Autodesk Inventor part; units mm, degrees
ref_plane "XZ Plane" through (0, 0, 0) normal (0, 1, 0) x (-1, 0, 0)
ref_plane "XY Plane" through (0, 0, 0) normal (0, 0, 1) x (1, 0, 0)
sketch "Sketch1" plane through (0, 0, 0) normal (0, 0, 1) x (1, 0, 0)
  line L0 (1, -23.75) -> (1, 25.75)
  line L1 (6, 30.75) -> (37, 30.75)
  line L2 (-37, -30.75) -> (-6, -30.75)
  arc A0 (-6, -30.75) -> (1, -23.75) centre (-6, -23.75) ccw
  arc A1 (6, 30.75) -> (1, 25.75) centre (6, 25.75) ccw
  line L3 (37, 32.75) -> (6, 32.75)
  arc A2 (6, 32.75) -> (-1, 25.75) centre (6, 25.75) ccw
  line L4 (-1, 25.75) -> (-1, -23.75)
  arc A3 (-6, -28.75) -> (-1, -23.75) centre (-6, -23.75) ccw
  line L5 (-6, -28.75) -> (-37, -28.75)
  line L6 (-37, -30.75) -> (-37, -28.75)
  line L7 (37, 30.75) -> (37, 32.75)
  point P0 (0, 0)
  dimension "d5" = 30.75
  dimension "d12" = 31
  dimension "d13" = 2
sketch "Sketch2" plane through (0, 0, 0) normal (1, 0, 0) x (0, 1, 0)
  line L0 (32.75, 0) -> (32.75, -1778.57)
  arc A0 (32.75, -1778.57) -> (55.2034, -1916.4389) centre (467.25, -1778.57) ccw
  line L1 (0, 0) -> (341.65, 0)
  line L2 (55.2034, -1916.4389) -> (194.6207, -2333.1133)
  dimension "d14" = 1778.57
  dimension "d17" = 161.5
  dimension "d18" = 439.38
  dimension "d28" = 434.5
sweep "Sweep1" add profiles "Sketch1" path "Sketch2" path curves L0 A0 L2
sketch "Sketch3" plane through (1, -23.75, 0) normal (1, 0, 0) x (0, 0, -1)
  line L0 (0, 49.5) -> (0, 0)
  line L1 (0, 0) -> (1778.57, 0)
  arc A0 (1778.57, 0) -> (1934.3666, 25.3731) centre (1778.57, 491) ccw
  line L2 (1934.3666, 25.3731) -> (2351.041, 164.7904)
  line L3 (2335.3345, 211.7324) -> (2351.041, 164.7904)
  line L4 (1918.66, 72.3151) -> (2335.3345, 211.7324)
  arc A1 (1778.57, 49.5) -> (1918.66, 72.3151) centre (1778.57, 491) ccw
  line L5 (0, 49.5) -> (1778.57, 49.5)
  line L6 (50, 83.8551) -> (50, -57.0573)
  line L7 (458.25, 83.8551) -> (458.25, -57.0573)
  line L8 (653.5, 83.8551) -> (653.5, -57.0573)
  circle A2 centre (1778.57, 491) radius 467.25
  line L9 (2343.1877, 188.2614) -> (1927.8399, 48.2348)
  line L10 (2020.5284, 268.8859) -> (2149.5287, -116.6554)
  line L11 (1818.57, 100.4548) -> (1818.57, -125.8263)
  line L12 (1936.5877, 18.7348) -> (1934.3666, 25.3731)
  line L13 (1778.57, -7) -> (1778.57, 0)
  circle A3 centre (2077.4777, 98.6823) radius 10
  circle A4 centre (1818.57, 25.4653) radius 10
  circle A5 centre (653.5, 23.75) radius 10
  circle A6 centre (458.25, 23.75) radius 10
  circle A7 centre (50, 23.75) radius 10
  point P0 (0, 23.75)
  dimension "d22" = 408.25
  dimension "d23" = 195.25
  dimension "d24" = 40
  dimension "d26" = 158.977
  dimension "d29" = 20
  dimension "d30" = 20
  dimension "d31" = 20
  dimension "d32" = 20
  dimension "d33" = 20
extrude "Extrusion1" cut sketch "Sketch3" against normal blind 10 contours A7 L6 | L6 A7 | A6 L7 | L7 A6 | A5 L8 | L8 A5 | A4 L11 A2 | A2 L11 A4 | L11 A4 A2 | A2 A4 L11 | A3 L9 L10 | L10 L9 A3 | A3 L9 L10 | L10 L9 A3
sketch "Sketch4" plane through (1, -23.75, 0) normal (1, 0, 0) x (0, 0, -1)
  line L0 (2335.3345, 211.7324) -> (2333.1133, 218.3707)
  line L1 (2333.1133, 218.3707) -> (2363.5204, -278.781)
  line L2 (1778.57, -7) -> (1778.57, 0)
  line L3 (2333.1133, 218.3707) -> (2448.2703, 211.7324)
  line L4 (2448.2703, 211.7324) -> (2363.5204, -278.781)
  point P0 (0, 23.75)
  dimension "d36" = 3.5
extrude "Extrusion2" cut sketch "Sketch4" along normal through all both and the other way through all
properties part number "AAD0001149621"
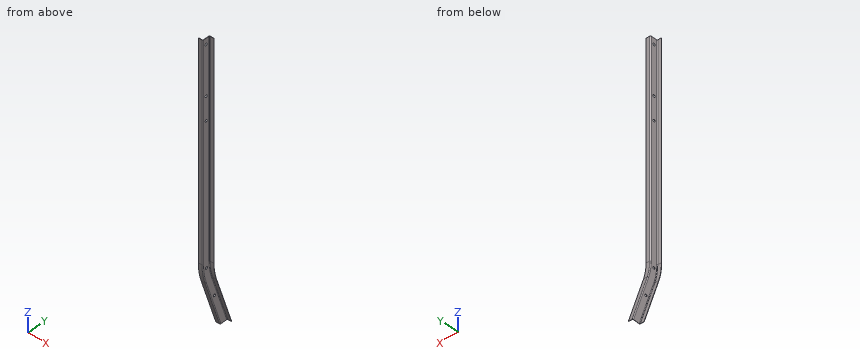
The model under review builds one solid part; all positions refer to its coordinate system, in mm. Round coordinates to 2 decimals unless told otherwise and drop trailing zeros. Order: outer loops, then holes, each group sorted by start corner. A loop starts at its lowest first (then second) coordinate and runs counter-clockwise, first axis right, second up. Notation, with made-up numbers: M -7,20.5 L 46,20.5 A30 cw 46,58.5 Z; hole C 15,-27.5 d3. An arc over 180 degrees is marked long. Use a Markdown table: item, result.
1) Consider section A-A (x = -20). Write out the cut boundary in (y, z), then the cut area to 3 significant figures.
Report:
| item | result |
|---|---|
| outline | M -30.75,-1778.57 A498 ccw -5.02,-1936.59 L 129,-2337.13 L 131.07,-2337 L -3.12,-1935.95 A496 cw -28.75,-1778.57 L -28.75,0 L -30.75,0 Z |
| area | 4,720 mm^2 |
2) Consider section B-B (z = -1437). Write out the cut boundary in (x, y).
Report:
| item | result |
|---|---|
| outline | M -37,-30.75 L -6,-30.75 A7 ccw 1,-23.75 L 1,25.75 A5 cw 6,30.75 L 37,30.75 L 37,32.75 L 6,32.75 A7 ccw -1,25.75 L -1,-23.75 A5 cw -6,-28.75 L -37,-28.75 Z |
3) Wall thickness on line 1 along Y through (x, z) = (-10, -450); line 2 along Y through (x, z) = (30, -471); line 3 along Y through (x, z) = (-0.05, -653.5): over which ranges is each line inside the solid? List them lowest first. Write a range as [from, to].
Report:
| item | result |
|---|---|
| line 1 | [-30.75, -28.75] |
| line 2 | [30.75, 32.75] |
| line 3 | [-27.44, -10], [10, 29.27] |
4) Insertion check: pin 1 (1 mm diameter, centred on x = 21, z = -1633.5, fed in from +Y); pin 2 (15.5 mm diameter, centred on x = -17.5, z = -618.5, fed in from +Y); pin 3 (18 mm diameter, centred on y = 0, z = -653.5, fed in from -X); pin 4 (15.5 mm diameter, centred on x = 26.5, z = -512.5, fed in from -Y). Each pin has a flat end and moves straight along its axis. Give the tip position at first contact, or say it passes through.
Report:
| item | result |
|---|---|
| pin 1 | y = 32.75 |
| pin 2 | y = -28.75 |
| pin 3 | through |
| pin 4 | y = 30.75 |
